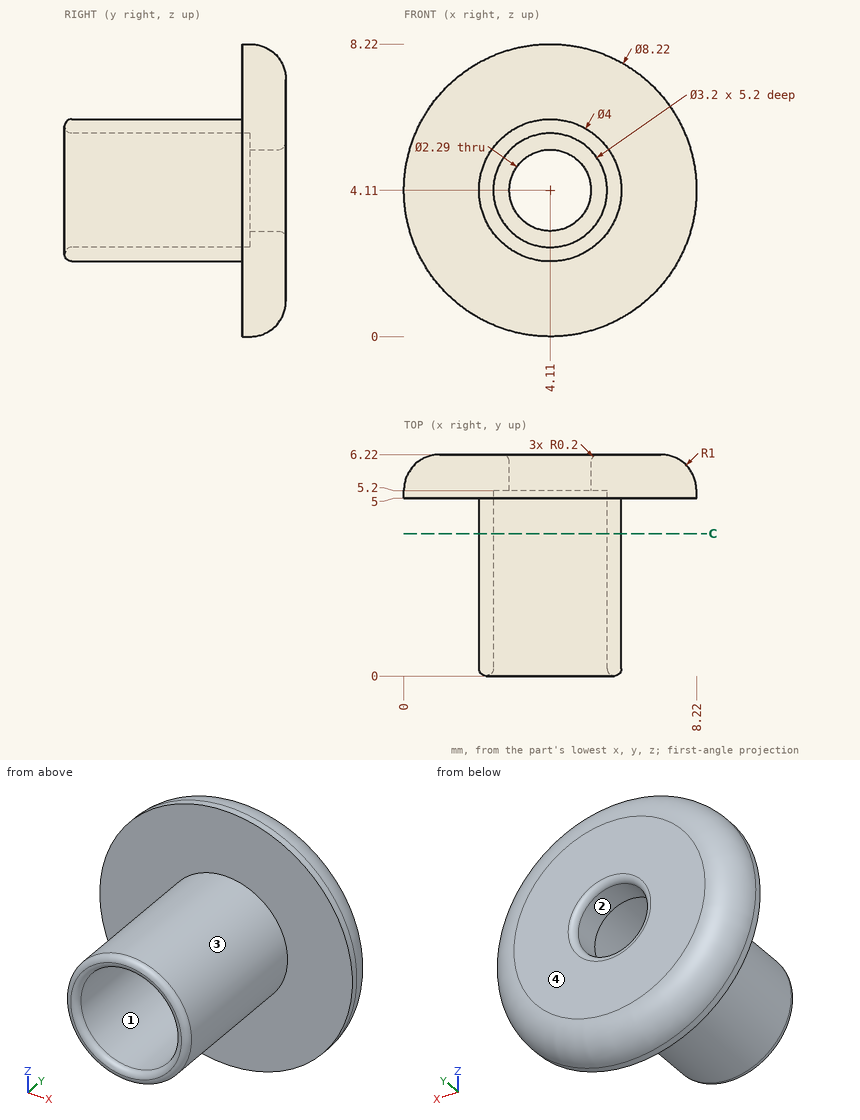
The drawing under review shows one solid part. Ordinate dimensions are in mm from its lowest x, y, z. Round coordinates to 2 decimals unless told otherwise and drop trailing zeros. Loops run counter-clockwise (first coordinate to the right, second up) from the corner with the lowest first, then second, coordinate; pieces in that order, holes last. Notation, with made-up numbers: (49.25, 34) - (77.25, 34) arc R3 cw to (77.25, 38) - close; hole circle Ø10 at (86.25, 79). An arc over 180 degrees is marked (long way). One line per question, with ' | ' between items.
1. Draft analysis for pull direction Z (two halves, no side actions). For the marked faces 1, 2, 3 and 4, state which applies: released by +Z, released by -Z, zero draft, split by the parting line, or undercut.
Results are:
face 1: undercut | face 2: undercut | face 3: split by the parting line | face 4: zero draft
2. Clearance check with flat-ended pins moving along their axes: P1, Ø4, axis at x = 7, z = 5, coming from the -Y side; P2, Ø1, axis at y = 3, z = 2.5, coming from the +X side (1 decimal). State where each tip first meets the part, or that it passes through.
Results are:
P1: stops at y = 0 | P2: stops at x = 5.8
3. We need section C-C, the plane y = 4. State the section outline as (x, z) points.
Results are:
outline: circle Ø4 at (4.11, 4.11); hole circle Ø3.2 at (4.11, 4.11)
4. For L1, parallel to Z at x = 4.11, y = 3.85; L2, parallel to Y at x = 6, z = 5.25; L3, parallel to Z at x = 3.75, y = 1.5, list the stretches that pass through material, from the lowest coordinate up. Write a range as [from, to].
Results are:
L1: z = [2.11, 2.51], [5.71, 6.11] | L2: y = [5, 6.22] | L3: z = [2.14, 2.55], [5.67, 6.08]
